Verification items for the finished model (mm, model axes). Round coordinates to 2 decimals unless told otherwise and drop trailing zeros. Write each loop counter-clockwise with the first axis right and the second up, starting at its lowest first coordinate (ties: lowest second). Pieces come first, ordered by that corner, then holes. Notation, with made-up numbers: M 89,49.5 L 113,49.5 A23 cw 113,87.5 Z; hole C 47,-22.5 d6. An arc over 180 degrees is marked long. Answer in a Markdown table with one row per item. Add a question column.
1. Go/stop test with flat-tipped pins: pin 1 Ø12.5 at (y, z) = (29.59, 0) entering from +X; pin 2 Ø5 at (x, z) = (113, 0) entering from -Y; pin 3 Ø4 at (x, y) = (109.5, 30) entering from -Z; pin 4 Ø4 at (x, y) = (111, 33.5) entering from +Z. Record where each tip stops, or that it passes through.
2. Material ranges on probe 1 along Y at (x, z) = (110.25, 0); probe 2 along Y at (x, z) = (115.25, 2.25); probe 3 along Z at (x, y) = (111.75, 34), recorded low to high.
3. Draft check along Z on faces 1 (the cylindrical face through (110.308, 21.695, 1.037)), 2 (the flat face through (103.67, 27, -8)). Enter one of: pulls with the +Z half, pulls with the -Z half, needs draft (parallel to the pull), parting line crosses it, or undercut.
4. Sectioned sample at C-C on x = 115. Record the cut outline in (y, z).
5. Sectioned sample at A-A on z = 0. Record the cut outline in (x, y).
6. Sectioned sample at B-B on x = 106.5. Record the cut outline in (y, z).
Autodesk Inventor part; units mm, degrees
ref_plane "YZ Plane" through (0, 0, 0) normal (1, 0, 0) x (0, 1, 0)
ref_plane "XZ Plane" through (0, 0, 0) normal (0, 1, 0) x (-1, 0, 0)
ref_plane "XY Plane" through (0, 0, 0) normal (0, 0, 1) x (1, 0, 0)
sketch "Sketch1" plane through (0, 0, 0) normal (0, 0, 1) x (1, 0, 0)
  arc A0 (103.6702, 18.7694) -> (117.1276, 18.7694) centre (110.3989, 29.5404) ccw
  line L0 (103.6702, 40.3608) -> (103.6702, 29.5898)
  line L1 (117.1276, 40.3608) -> (117.1276, 29.5898)
  line L2 (95.2163, 29.5898) -> (125.5815, 29.5898)
  arc A1 (117.1276, 40.3608) -> (103.6702, 40.3608) centre (110.3989, 29.5898) ccw
  point P0 (0, 0)
  point P1 (110.3989, 16.8404)
  dimension "d44" = 21.6408
  dimension "d45" = 12.7
  dimension "d46" = 12.7
revolve "Revolution1" add sketch "Sketch1" angle 360 about axis through (95.2163, 29.5898, 0) along (1, 0, 0)
sketch "Sketch2" plane through (117.1276, 29.5898, 0) normal (1, 0, 0) x (0, 0, -1)
  circle A0 centre (0, 0) radius 10.771
  point P0 (0, -29.5898)
hole "Hole1" at (117.1276, 29.5898, 0) direction (-1, 0, 0) diameter 15.9258 depth 25.4 tip angle 118
chamfer "Chamfer1" distance 0.254 angle 45 2 edges at (117.1276, 29.5898, 7.9629) (103.6702, 29.5898, 7.9629)
equation "\"d45\" = d46"
properties part number "1410P"
Geometry check:
| question | item | result |
|---|---|---|
| 1 | pin 1 | passes through |
| 1 | pin 2 | stops at y = 16.89 |
| 1 | pin 3 | stops at z = -12.7 |
| 1 | pin 4 | stops at z = 12.55 |
| 2 | probe 1 | y = 16.89 to 21.63, 37.55 to 42.29 |
| 2 | probe 2 | y = 18.07 to 21.95, 37.23 to 41.11 |
| 2 | probe 3 | z = -11.83 to -6.63, 6.63 to 11.83 |
| 3 | face 1 | undercut |
| 3 | face 2 | needs draft |
| 4 | outline | C 29.59,0 d23.67; hole C 29.59,0 d15.93 |
| 5 | outline | M 103.67,18.82 A12.7 ccw 117.13,18.82 L 117.13,21.37 L 116.87,21.63 L 103.92,21.63 L 103.67,21.37 Z; M 103.67,37.81 L 103.92,37.55 L 116.87,37.55 L 117.13,37.81 L 117.13,40.36 A12.7 ccw 103.67,40.36 Z |
| 6 | outline | C 29.59,0 d24.17; hole C 29.59,0 d15.93 |
